from build123d import *

# Parameters (mm, degrees)
SKETCH1_W           = 42
SKETCH1_H           = 15
BOSS_EXTRUDE1_DEPTH = 9.5
CUT_EXTRUDE1_REACH  = 11.5
SKETCH2_R           = 6
SKETCH4_R           = 1.9
CUT_EXTRUDE3_DEPTH  = 2
SKETCH5_R           = 2.05
CUT_EXTRUDE4_DEPTH  = 5
SKETCH6_R           = 0.95
CUT_EXTRUDE5_DEPTH  = 3
FILLET1_R           = 7
SKETCH7_W           = 6
SKETCH7_H           = 9.5
CUT_EXTRUDE6_DEPTH  = 3


with BuildPart() as part:
    # Sketch1 → Boss-Extrude1 (new body)
    with BuildSketch(Plane(origin=(0, 0, 0), x_dir=(1, 0, 0), z_dir=(0, 1, 0))):
        with Locations((21, 7.5)):
            Rectangle(SKETCH1_W, SKETCH1_H)
    extrude(amount=-BOSS_EXTRUDE1_DEPTH)

    # Sketch2 → Cut-Extrude1 (cut, up to next)
    with BuildSketch(Plane(origin=(0, 0, 0), x_dir=(1, 0, 0), z_dir=(0, 1, 0)), mode=Mode.PRIVATE) as cut_extrude1_sk1:
        with Locations((21, 7.5)):
            Circle(SKETCH2_R)
    cut_extrude1_tool1 = extrude(cut_extrude1_sk1.sketch, amount=-CUT_EXTRUDE1_REACH, mode=Mode.PRIVATE) & part.part
    add(cut_extrude1_tool1.solids().sort_by_distance((21, 0, -7.5))[0], mode=Mode.SUBTRACT)

    # Sketch4 → Cut-Extrude3 (cut)
    with BuildSketch(Plane(origin=(0, 0, 0), x_dir=(1, 0, 0), z_dir=(0, 1, 0))):
        with Locations((4.5, 7.5)):
            Circle(SKETCH4_R)
        with Locations((37.5, 7.5)):
            Circle(SKETCH4_R)
    extrude(amount=-CUT_EXTRUDE3_DEPTH, mode=Mode.SUBTRACT)

    # Sketch5 → Cut-Extrude4 (cut)
    with BuildSketch(Plane(origin=(0, -9.5, 0), x_dir=(-1, 0, 0), z_dir=(0, -1, 0))):
        with Locations((-37.5, 7.5)):
            Circle(SKETCH5_R)
        with Locations((-4.5, 7.5)):
            Circle(SKETCH5_R)
    extrude(amount=-CUT_EXTRUDE4_DEPTH, mode=Mode.SUBTRACT)

    # Sketch6 → Cut-Extrude5 (cut)
    with BuildSketch(Plane(origin=(0, -2, 0), x_dir=(1, 0, 0), z_dir=(0, 1, 0))):
        with Locations((4.5, 7.5)):
            Circle(SKETCH6_R)
        with Locations((37.5, 7.5)):
            Circle(SKETCH6_R)
    extrude(amount=-CUT_EXTRUDE5_DEPTH, mode=Mode.SUBTRACT)

    # Fillet1
    fillet1_edges = [part.edges().sort_by_distance(p)[0] for p in [
        (0, -4.75, -15),
        (42, -4.75, -15),
        (42, -4.75, 0),
        (0, -4.75, 0),
    ]]
    fillet(fillet1_edges, radius=FILLET1_R)

    # Sketch7 → Cut-Extrude6 (cut)
    with BuildSketch(Plane(origin=(0, 0, -15), x_dir=(-1, 0, 0), z_dir=(0, 0, -1))):
        with Locations((-21, -4.75)):
            Rectangle(SKETCH7_W, SKETCH7_H)
    extrude(amount=-CUT_EXTRUDE6_DEPTH, mode=Mode.SUBTRACT)


solid = part.part
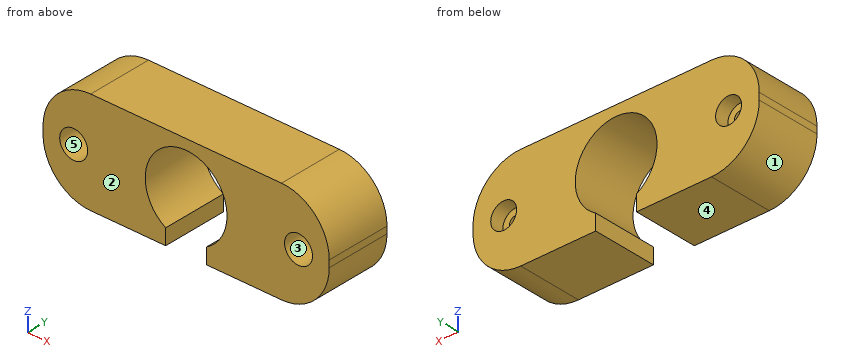
Could you check a few things on this model? Use its own coordinates, in mm. Face numbers are marked on the shaded views. A direction names the side the tool comes from. Coordinates: 2 decimals unless noted, no trailing zeros. Loops run counter-clockwise (first coordinate to the right, second up) from the corner with the lowest first, then second, coordinate; pieces in that order, holes last.
1. Imagine slicing it at D-D (x = 37.5). Please give me the cut outline in (y, z), and give its area (3 significant figures).
2. Imagine slicing it at B-B (z = -7.5). Give the number of separate pieces and of enclosed holes in the cut face, and give its area (3 significant figures).
3. Imagine slicing it at A-A (y = -1.5). Please give me the cut outline in (x, z), and give its area (3 significant figures).
4. I need wall thicknesses on L1, parallel to X at y = -8.5, z = -8.75; L2, parallel to Z at x = 21, y = -6.75; L3, parallel to X at y = -8, z = -4.5. Which ranges of each line are inside material? Lowest first, please.
5. For P1, Ø1, axis at y = -4.5, z = -3.5, coming from the +X side; P2, Ø2.5, axis at x = 4.5, z = -7.5, coming from the +Y side; P3, Ø2, axis at x = 5, z = -8, coming from the -Y side, each with a flat end and sliding along its axis, tell me the tip position at first contact or that it passes through.
6. For the marked faces 4 and 5, which set-ups out of +Z, -Z, +X, -X, +Y, -Y let a thin tool reach every point of the face, with its end or its side?
7. Imagine slicing it at C-C (z = -13.25). Please give me the cut outline in (x, y).
8. We'd pull the mould along X, two halves only. Please class the marked faces 1, 2 and 3: released by +X, released by -X, zero draft, split by the parting line, or undercut.
Computed values:
1. outline: (-9.5, -14.54) - (0, -14.54) - (0, -9.4) - (-2, -9.4) - (-2, -8.45) - (-4.5, -8.45) - (-4.5, -9.55) - (-9.5, -9.55) - close; (-9.5, -5.45) - (-4.5, -5.45) - (-4.5, -6.55) - (-2, -6.55) - (-2, -5.6) - (0, -5.6) - (0, -0.46) - (-9.5, -0.46) - close
1. area: 101 mm2
2. separate pieces: 4
2. enclosed holes: 0
2. area: 219 mm2
3. outline: (0, -8) arc R7 ccw to (7, -15) - (18, -15) - (18, -12.7) arc R6 cw (long way) to (24, -12.7) - (24, -15) - (35, -15) arc R7 ccw to (42, -8) - (42, -7) arc R7 ccw to (35, 0) - (7, 0) arc R7 ccw to (0, -7) - close; hole circle Ø3.8 at (4.5, -7.5); hole circle Ø3.8 at (37.5, -7.5)
3. area: 442 mm2
4. L1: x = 0.04 to 2.88, 6.12 to 15.13, 26.87 to 35.88, 39.12 to 41.96
4. L2: z = -1.5 to 0
4. L3: x = 0.46 to 15.8, 26.2 to 41.54
5. P1: stops at x = 41.32
5. P2: stops at y = -2
5. P3: stops at y = -4.5
6. face 4: -Z, +X, -X, +Y, -Y
6. face 5: -Y
7. outline: (2.37, -9.5) - (18, -9.5) - (18, 0) - (2.37, 0) - close; (24, -9.5) - (39.63, -9.5) - (39.63, 0) - (24, 0) - close
8. face 1: released by -X
8. face 2: zero draft
8. face 3: undercut
